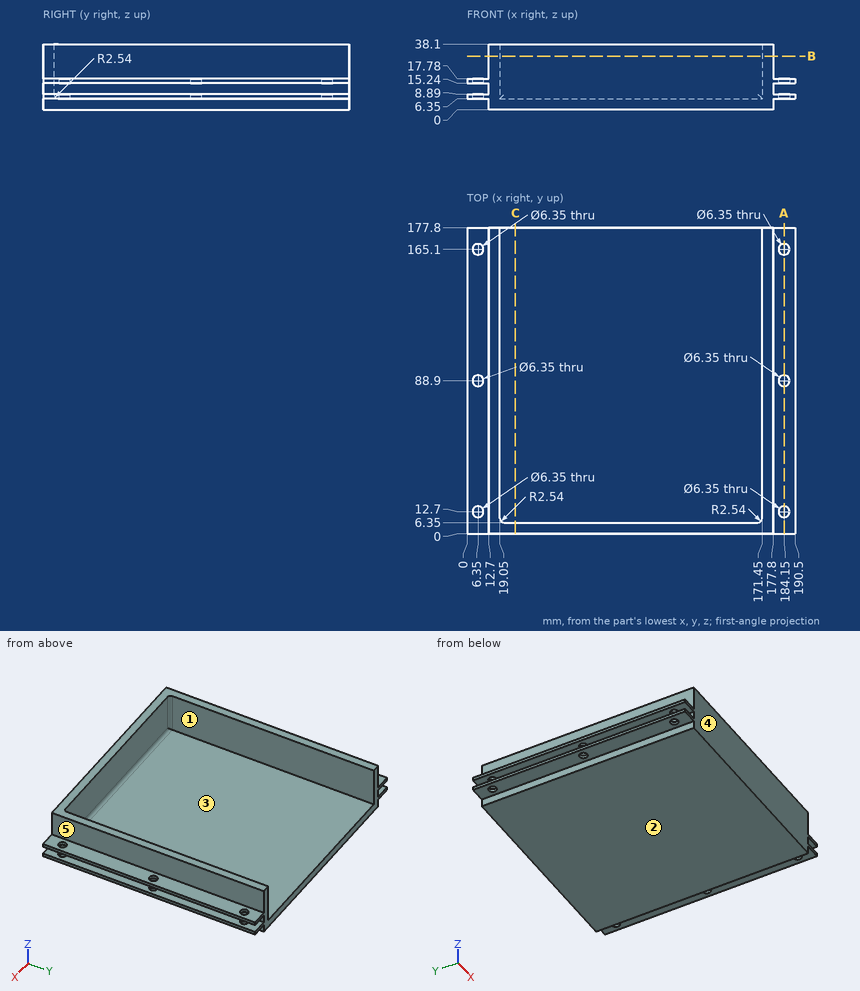
Drawing for the job (mm, zero at the part's lowest x, y, z). A direction names the side the tool comes from. Give positions to 0.01 mm unless a question says otherwise; leave off trailing zeros. Write each loop counter-clockwise with the first axis right and the second up, starting at its lowest first coordinate (ties: lowest second). Pieces come first, ordered by that corner, then holes. Notation, with made-up numbers: (-12, 77.5) -> (12, 77.5) arc R20 ccw to (12, 90.5) -> close; hole circle Ø3 at (45.5, 25). An arc over 180 degrees is marked (long way). Put each result on its own line as item: value. Start each with the question number.
Item 1: Cut at B-B (z = 31). List the corners of the cut face in (x, y), then the cut area to 3 significant figures.
Item 2: Pin check, flat tips, straight feed: pin 1 Ø7.5 at (x, y) = (184.15, 12.7) entering from +Z; pin 2 Ø6.5 at (x, y) = (9, 128.5) entering from -Z; pin 3 Ø6 at (y, z) = (124.5, 26.5) entering from -X; pin 4 Ø8 at (y, z) = (139, 16) entering from -X. Stop position of each tip, or through.
Item 3: Which spindle directions (+Z, -Z, +X, -X, +Y, -Y) get a long thin tool onto all of the face, cutting with end or side? Do the marked faces 1 and 2. Say none if no direction does.
Item 4: Wall check: L1, parallel to X at y = 165, z = 17; L2, parallel to Y at x = 184.15, z = 7.75 (3 decimals); L3, parallel to X at y = 18.5, z = 33.5. Give the ranges that are in metal, low to high. Write a range as [from, to].
Item 5: Cut at C-C (x = 28). List the corners of the cut face in (y, z), then the cut area to 3 significant figures.
Item 6: Pull direction X, two halves, no side cores. Call the marked faces 3, 4 and 5: pulls with the +X half, pulls with the -X half, needs draft (parallel to the pull), parting line crosses it, or undercut.
Item 7: Cut at A-A (x = 184.15). State how many separate pieces and enclosed holes the cut face has, then the cut area to 3 significant figures.
Answer list:
1. outline: (12.7, 0) -> (177.8, 0) -> (177.8, 177.8) -> (171.45, 177.8) -> (171.45, 8.89) arc R2.54 cw to (168.91, 6.35) -> (21.59, 6.35) arc R2.54 cw to (19.05, 8.89) -> (19.05, 177.8) -> (12.7, 177.8) -> close
1. area: 3,230 mm2
2. pin 1: stops at z = 17.78
2. pin 2: stops at z = 6.35
2. pin 3: stops at x = 12.7
2. pin 4: stops at x = 0
3. face 1: +Z, +Y
3. face 2: -Z, +X, -X, +Y, -Y
4. L1: x = [0, 3.18], [9.52, 19.05], [171.45, 180.98], [187.32, 190.5]
4. L2: y = [0, 9.525], [15.875, 85.725], [92.075, 161.925], [168.275, 177.8]
4. L3: x = [12.7, 19.05], [171.45, 177.8]
5. outline: (0, 0) -> (177.8, 0) -> (177.8, 6.35) -> (8.89, 6.35) arc R2.54 cw to (6.35, 8.89) -> (6.35, 38.1) -> (0, 38.1) -> close
5. area: 1,330 mm2
6. face 3: undercut
6. face 4: needs draft
6. face 5: pulls with the +X half
7. separate pieces: 8
7. enclosed holes: 0
7. area: 806 mm2
